The drawing under review shows one solid part. Ordinate dimensions are in mm from its lowest x, y, z. Coordinates: 2 decimals unless noted, no trailing zeros. Order: outer loops, then holes, each group sorted by start corner. A loop starts at its lowest first (then second) coordinate and runs counter-clockwise, first axis right, second up. Notation, with made-up numbers: (42.25, 14.25) - (80.25, 14.25) arc R15 ccw to (80.25, 21.25) - close; hole circle Ø10 at (58, 4). An arc over 180 degrees is marked (long way). Write item = value, one per line. Start each with the question number.
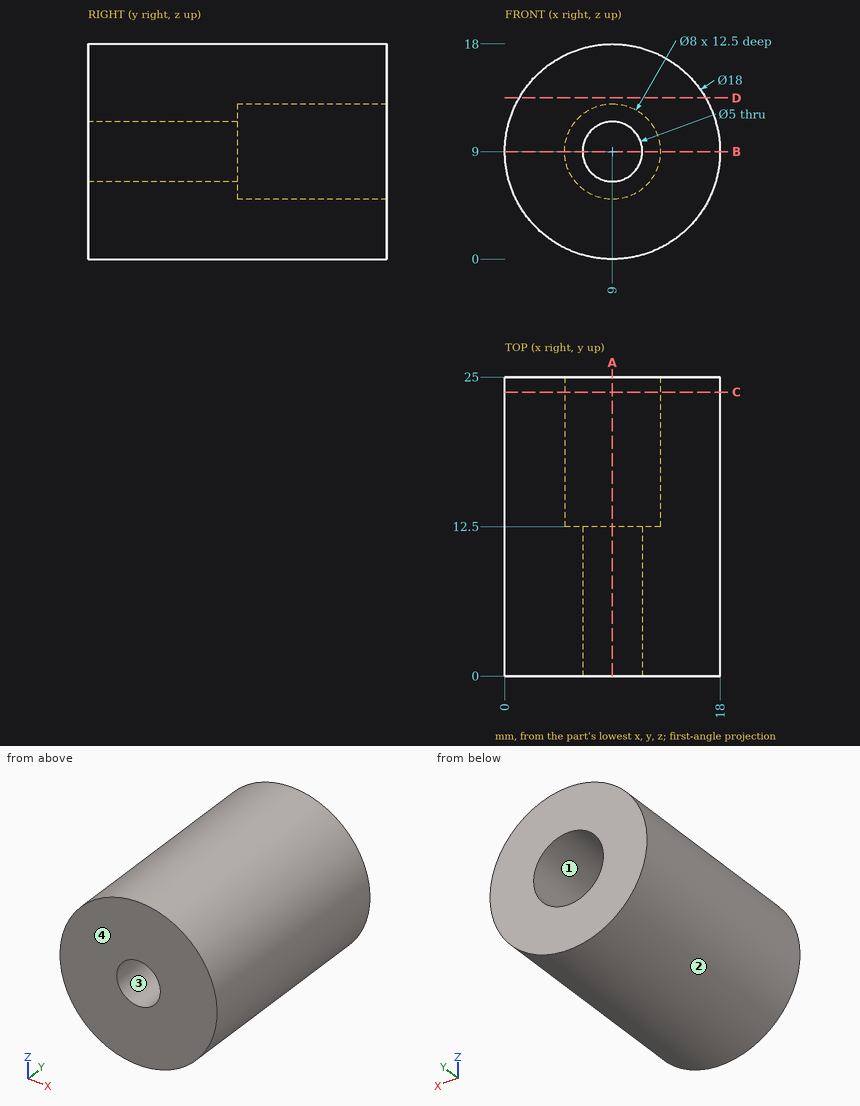
Item 1: For line 1 (X direction, y = 18, z = 9); line 2 (X direction, y = 9.5, z = 9); line 3 (Z direction, x = 8.25, y = 21.5), list the stretches that pass through material, from the lowest coordinate up.
Item 2: Add section A-A on x = 9. Give the boundary of the cut face in (y, z).
Item 3: Add section D-D on z = 13.5. Give the boundary of the cut face in (x, y), plus the area to 3 significant figures.
Item 4: Mouldability with a two-part tool opening along Z and no side actions: class the marked faces 1, 2, 3 and 4 as +Z half, -Z half, draft (parallel to the pull), parting line (faces both ways), or undercut.
Item 5: Add section B-B on z = 9. Give the boundary of the cut face in (x, y), plus the area to 4 significant figures.
Item 6: Add section C-C on y = 23.75. Give the boundary of the cut face in (x, z), plus the area to 3 significant figures.
Item 7: For P1, Ø8, axis at x = 2, y = 21, coming from the +Z side; P2, Ø5, axis at x = 11.5, z = 9, coming from the -Y side; P3, Ø1.5, axis at y = 13.5, z = 13.5, coming from the +X side; P4, Ø1.5, axis at x = 13.5, y = 12, coming from the +Z side, all flat-tipped, find the tip position at first contact; note any pin that passes through.
Worked out:
q1.line_1 = 0 to 5, 13 to 18
q1.line_2 = 0 to 6.5, 11.5 to 18
q1.line_3 = 0.03 to 5.07, 12.93 to 17.97
q2.outline = (0, 0) - (25, 0) - (25, 5) - (12.5, 5) - (12.5, 6.5) - (0, 6.5) - close; (0, 11.5) - (12.5, 11.5) - (12.5, 13) - (25, 13) - (25, 18) - (0, 18) - close
q3.outline = (1.21, 0) - (16.79, 0) - (16.79, 25) - (1.21, 25) - close
q3.area = 390 mm2
q4.face_1 = undercut
q4.face_2 = parting line
q4.face_3 = undercut
q4.face_4 = draft
q5.outline = (0, 0) - (6.5, 0) - (6.5, 12.5) - (5, 12.5) - (5, 25) - (0, 25) - close; (11.5, 0) - (18, 0) - (18, 25) - (13, 25) - (13, 12.5) - (11.5, 12.5) - close
q5.area = 287.5 mm2
q6.outline = circle Ø18 at (9, 9); hole circle Ø8 at (9, 9)
q6.area = 204 mm2
q7.P1 = 17.49
q7.P2 = 0
q7.P3 = 17.18
q7.P4 = 17.18
